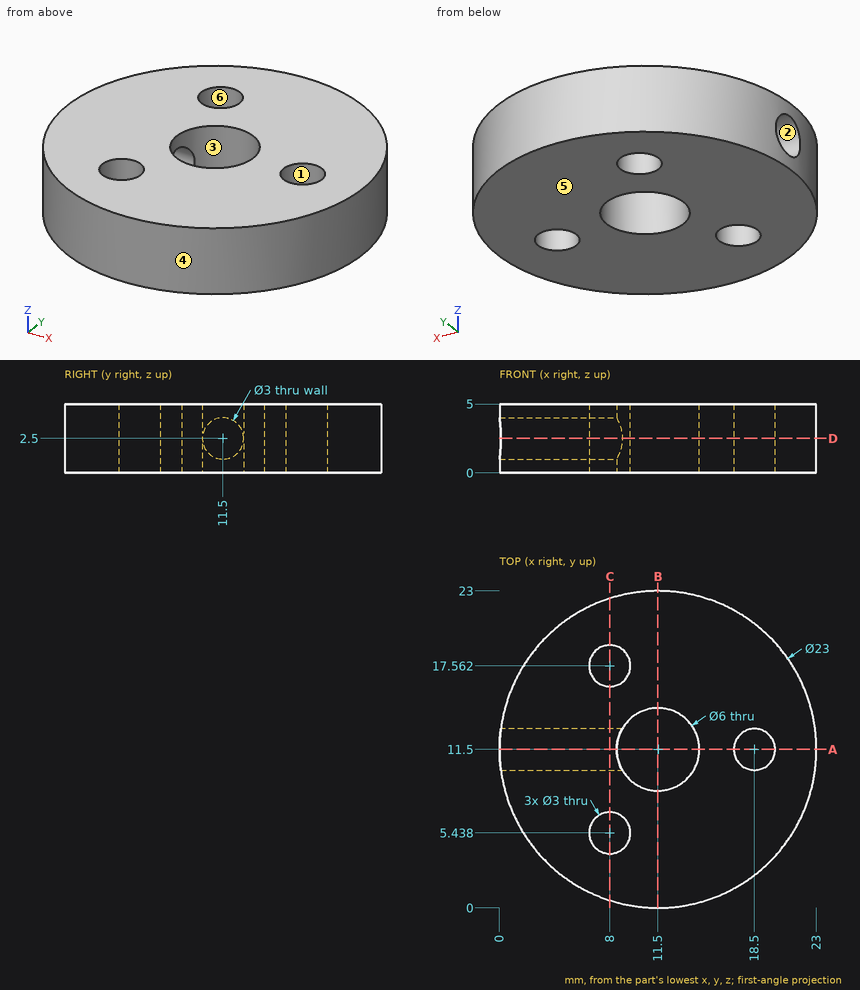
Input: dimensioned drawing with shaded views. Units: mm. Origin: part minimum x, y, z. A direction names the side the tool comes from. Coordinates: 2 decimals unless noted, no trailing zeros. Order: outer loops, then holes, each group sorted by start corner. A loop starts at its lowest first (then second) coordinate and runs counter-clockwise, first axis right, second up.
1. Cut plane B-B, the plane x = 11.5. Return loops of the section in (y, z).
Checked values:
outline: (0, 0) - (8.5, 0) - (8.5, 5) - (0, 5) - close; (14.5, 0) - (23, 0) - (23, 5) - (14.5, 5) - close
2. Ray query, line 1 along Y through (x, z) = (8, 1.8) (1 decimal); line 2 along Y through (x, z) = (8, 2.05) (1 decimal); line 3 along Z through (x, y) = (6.5, 11.25). Return the intervals inside material, ascending.
Checked values:
line 1: y = 0.5 to 3.9, 6.9 to 10.2, 12.8 to 16.1, 19.1 to 22.5
line 2: y = 0.5 to 3.9, 6.9 to 10.1, 12.9 to 16.1, 19.1 to 22.5
line 3: z = 0 to 1.02, 3.98 to 5
3. Cut plane C-C, the plane x = 8. Return loops of the section in (y, z).
Checked values:
outline: (0.55, 0) - (3.94, 0) - (3.94, 5) - (0.55, 5) - close; (6.94, 0) - (16.06, 0) - (16.06, 5) - (6.94, 5) - close; (19.06, 0) - (22.45, 0) - (22.45, 5) - (19.06, 5) - close; hole circle Ø3 at (11.5, 2.5)
4. Draft query along X for the marked faces 3, 4, 5 and 6. Return one class per face: +X half, -X half, draft (parallel to the pull), parting line (faces both ways), or undercut.
Checked values:
face 3: undercut
face 4: parting line
face 5: draft
face 6: undercut
5. Contact query for flat-ended pins moving along their axis: P1, Ø3, axis at y = 20, z = 1, coming from the +X side; P2, Ø1, axis at y = 11.5, z = 2, coming from the -X side; P3, Ø1.8, axis at y = 11.5, z = 2.5, coming from the -X side. Output: stop coordinate, or through.
Checked values:
P1: stops at x = 20.62
P2: stops at x = 14.46
P3: stops at x = 14.36
6. Cut plane D-D, the plane z = 2.5. Return loops of the section in (x, y).
Checked values:
outline: (0.1, 10) arc R11.5 ccw (long way) to (0.1, 13) - (8.9, 13) arc R3 cw (long way) to (8.9, 10) - close; hole circle Ø3 at (8, 5.44); hole circle Ø3 at (8, 17.56); hole circle Ø3 at (18.5, 11.5)
7. Access query for the marked faces 1 and 2. Directions: +Z, -Z, +X, -X, +Y, -Y. A direction counts if a zero-diameter tool reaches every point of the face in a straight line with its end or side. Return the directions, or none.
Checked values:
face 1: +Z, -Z
face 2: -X
8. Cut plane A-A, the plane y = 11.5. Return loops of the section in (x, z), plus the area to 3 significant figures.
Checked values:
outline: (0, 0) - (8.5, 0) - (8.5, 1) - (0, 1) - close; (0, 4) - (8.5, 4) - (8.5, 5) - (0, 5) - close; (14.5, 0) - (17, 0) - (17, 5) - (14.5, 5) - close; (20, 0) - (23, 0) - (23, 5) - (20, 5) - close
area: 44.5 mm2
